Work out the finished part from the listing and answer in its coordinate system (mm). Face numbers are marked on the shaded views. Give positions to 0.01 mm unless a question says otherwise; leave off trailing zeros. Loops run counter-clockwise (first coordinate to the right, second up) from the corner with the lowest first, then second, coordinate; pieces in that order, holes last.
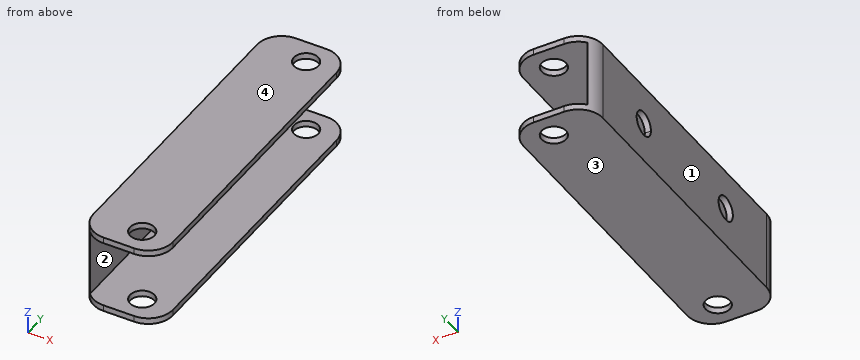
from build123d import *

# Parameters (mm, degrees)
F2_DEPTH    = 135
F1_R        = 5
F3_DEPTH    = 46
F4_T1_DEPTH = 52.5
F4_T3_DEPTH = 52.5
F4_T5_DEPTH = 82.5
F7_DEPTH    = 25


# Not quite as in the source:
# - a fillet or chamfer that OpenCascade refuses, or shapes differently, is made with other operations: its cross-section is extruded or revolved along the edge and cut away or added


with BuildPart() as f2:
    # F0 (on Front) → F2 (new body)
    with BuildSketch(Plane.XZ):
        Polygon((-74.9858543277, 32.5), (-74.9858543277, 0), (-42.4858543277, 0), (-42.4858543277, 2.5), (-72.4858543277, 2.5), (-72.4858543277, 30), (-42.4858543277, 30), (-42.4858543277, 32.5), align=None)
    extrude(amount=F2_DEPTH)

    # F1 (on Top) → F3 (cut)
    with BuildSketch(Plane.XY):
        with Locations((-54.9858543277, -260)):
            Circle(F1_R)
        with Locations((-54.9858543277, -125)):
            Circle(F1_R)
        with Locations((-54.9858543277, -10)):
            Circle(F1_R)
    extrude(amount=F3_DEPTH, mode=Mode.SUBTRACT)

    # F4: fillet of radius 10 on 6 edges, made by hand

    # F4_s2 → F4_t1 (cut)
    with BuildSketch(Plane.XY.offset(-25)):
        with BuildLine():
            ThreePointArc((-52.4858543277, 0), (-45.4147865158, -2.9289321881), (-42.4858543277, -10))
            Line((-42.4858543277, -10), (-42.4858543277, 0))
            Line((-42.4858543277, 0), (-52.4858543277, 0))
        make_face()
        with BuildLine():
            ThreePointArc((-52.4858543277, -135), (-45.4147865158, -132.0710678119), (-42.4858543277, -125))
            Line((-42.4858543277, -125), (-42.4858543277, -135))
            Line((-42.4858543277, -135), (-52.4858543277, -135))
        make_face()
    extrude(amount=F4_T1_DEPTH, mode=Mode.SUBTRACT)

    # F4_s4 → F4_t3 (cut)
    with BuildSketch(Plane.XY.offset(5)):
        with BuildLine():
            ThreePointArc((-42.4858543277, -10), (-45.4147865158, -2.9289321881), (-52.4858543277, 0))
            Line((-52.4858543277, 0), (-42.4858543277, 0))
            Line((-42.4858543277, 0), (-42.4858543277, -10))
        make_face()
        with BuildLine():
            ThreePointArc((-42.4858543277, -125), (-45.4147865158, -132.0710678119), (-52.4858543277, -135))
            Line((-52.4858543277, -135), (-42.4858543277, -135))
            Line((-42.4858543277, -135), (-42.4858543277, -125))
        make_face()
    extrude(amount=F4_T3_DEPTH, mode=Mode.SUBTRACT)

    # F4_s6 → F4_t5 (cut)
    with BuildSketch(Plane.XY.offset(-25)):
        with BuildLine():
            ThreePointArc((-64.9858543277, 0), (-72.0569221395, -2.9289321881), (-74.9858543277, -10))
            Line((-74.9858543277, -10), (-74.9858543277, 0))
            Line((-74.9858543277, 0), (-64.9858543277, 0))
        make_face()
        with BuildLine():
            ThreePointArc((-64.9858543277, -135), (-72.0569221395, -132.0710678119), (-74.9858543277, -125))
            Line((-74.9858543277, -125), (-74.9858543277, -135))
            Line((-74.9858543277, -135), (-64.9858543277, -135))
        make_face()
    extrude(amount=F4_T5_DEPTH, mode=Mode.SUBTRACT)

    # F6 (on offset) → F7 (cut)
    with BuildSketch(Plane(origin=(-74.9858543277, 0, 0), x_dir=(0, -1, 0), z_dir=(-1, 0, 0))):
        with BuildLine():
            Line((38.75, 16.25), (43.75, 16.25))
            ThreePointArc((43.75, 16.25), (35.2144660941, 19.7855339059), (38.75, 11.25))
            Line((38.75, 11.25), (38.75, 16.25))
        make_face()
        with BuildLine():
            ThreePointArc((38.75, 11.25), (42.2855339059, 12.7144660941), (43.75, 16.25))
            Line((43.75, 16.25), (38.75, 16.25))
            Line((38.75, 16.25), (38.75, 11.25))
        make_face()
        with BuildLine():
            ThreePointArc((101.25, 16.25), (96.25, 21.25), (91.25, 16.25))
            ThreePointArc((91.25, 16.25), (96.25, 11.25), (101.25, 16.25))
        make_face()
    extrude(amount=-F7_DEPTH, mode=Mode.SUBTRACT)


solid = f2.part
Item 1: Find section A-A, the plane y = -96.25. Write down the section's boundary in (x, z).
Item 2: Consider line 1 (Z direction, x = -50, y = -68.5); line 2 (X direction, y = -33, z = 16.5); line 3 (X direction, y = -125, z = 1). Determine where each line is inside the solid, lowest interval first.
Item 3: Find section C-C, the plane y = -81. Write down the section's boundary in (x, z).
Item 4: Determine the mould class of the marked faces 1, 2, 3 and 4 for opening direction Z: released by +Z, released by -Z, zero draft, split by the parting line, or undercut.
Item 5: Find section B-B, the plane x = -54. Write down the section's boundary in (y, z), plus the area to 3 significant figures.
Item 6: Find section D-D, the plane z = 19. Write down the section's boundary in (x, y), plus the area to 3 significant figures.
Item 7: Flat-ended cylindrical pins translate along their axes: pin 1 Ø14 at (y, z) = (-48, 20.5) entering from +X; pin 2 Ø3 at (x, y) = (-68, -80.5) entering from -Z; pin 3 Ø6 at (y, z) = (-96.25, 16.25) entering from +X. Find the tip coordinate at first contact, or state that the pin passes through.
Ans:
1. outline: (-74.99, 0) - (-42.49, 0) - (-42.49, 2.5) - (-72.49, 2.5) - (-72.49, 11.25) - (-74.99, 11.25) - close; (-74.99, 21.25) - (-72.49, 21.25) - (-72.49, 30) - (-42.49, 30) - (-42.49, 32.5) - (-74.99, 32.5) - close
2. line 1: z = 0 to 2.5, 30 to 32.5
2. line 2: x = -74.99 to -72.49
2. line 3: x = -74.99 to -59.99, -49.99 to -42.49
3. outline: (-74.99, 0) - (-42.49, 0) - (-42.49, 2.5) - (-72.49, 2.5) - (-72.49, 30) - (-42.49, 30) - (-42.49, 32.5) - (-74.99, 32.5) - close
4. face 1: zero draft
4. face 2: undercut
4. face 3: released by -Z
4. face 4: released by +Z
5. outline: (-135, 0) - (-129.9, 0) - (-129.9, 2.5) - (-135, 2.5) - close; (-135, 30) - (-129.9, 30) - (-129.9, 32.5) - (-135, 32.5) - close; (-120.1, 0) - (-14.9, 0) - (-14.9, 2.5) - (-120.1, 2.5) - close; (-120.1, 30) - (-14.9, 30) - (-14.9, 32.5) - (-120.1, 32.5) - close; (-5.1, 0) - (0, 0) - (0, 2.5) - (-5.1, 2.5) - close; (-5.1, 30) - (0, 30) - (0, 32.5) - (-5.1, 32.5) - close
5. area: 577 mm2
6. outline: (-74.99, -125) arc R10 ccw to (-72.49, -131.61) - (-72.49, -100.43) - (-74.99, -100.43) - close; (-74.99, -92.07) - (-72.49, -92.07) - (-72.49, -42.93) - (-74.99, -42.93) - close; (-74.99, -34.57) - (-72.49, -34.57) - (-72.49, -3.39) arc R10 ccw to (-74.99, -10) - close
6. area: 268 mm2
7. pin 1: stops at x = -72.49
7. pin 2: stops at z = 0
7. pin 3: passes through
